from build123d import *

# Parameters (mm, degrees)
SM_BASE_FLANGE_1_DEPTH     = 1.5
SKETCH_6_R                 = 6.5
CUT_EXTRUDE_1_DEPTH        = 10
PATTERN_LINEAR_1_COUNT     = 2
PATTERN_LINEAR_1_PITCH     = 20
PATTERN_LINEAR_1_COL_COUNT = 2
PATTERN_LINEAR_1_COL_PITCH = 20
CHAMFER_1_SIZE             = 10


# Sheet-metal steps are written as plain solids
with BuildPart() as part:
    # Sketch 1 → Базовая кромка1 (new body)
    with BuildSketch(Plane.XY):
        Polygon((-50, 0), (50, 0), (50, 30), (0, 80), (-50, 30), align=None)
    extrude(amount=-SM_BASE_FLANGE_1_DEPTH)

    # Эскиз6 → Вырез-Вытянуть1 (cut)
    with BuildSketch(Plane.XY):
        with Locations((0, 32.623845661)):
            Circle(SKETCH_6_R)
    cut_extrude_1 = extrude(amount=-CUT_EXTRUDE_1_DEPTH, mode=Mode.SUBTRACT)

    # Линейный массив1: Вырез-Вытянуть1 ×2
    with Locations(*[(-i * PATTERN_LINEAR_1_PITCH, 0, 0) for i in range(1, PATTERN_LINEAR_1_COUNT)]):
        add(cut_extrude_1, mode=Mode.SUBTRACT)

    # Линейный массив1 col: Вырез-Вытянуть1 ×2
    with Locations(*[(i * PATTERN_LINEAR_1_COL_PITCH, 0, 0) for i in range(1, PATTERN_LINEAR_1_COL_COUNT)]):
        add(cut_extrude_1, mode=Mode.SUBTRACT)

    # Фаска1
    chamfer_1_edges = [part.edges().sort_by_distance(p)[0] for p in [
        (0, 80, -0.75),
    ]]
    chamfer(chamfer_1_edges, length=CHAMFER_1_SIZE)


solid = part.part
Geometry check sheet. Reference: the model listing, model coordinates, mm. Round coordinates to 2 decimals unless told otherwise and drop trailing zeros. Write each loop counter-clockwise with the first axis right and the second up, starting at its lowest first coordinate (ties: lowest second). Pieces come first, ordered by that corner, then holes. Notation, with made-up numbers: (2, -29.5) -> (50, -29.5) arc R34 cw to (50, 8.5) -> close; hole circle Ø1 at (72.25, -12.75). An arc over 180 degrees is marked (long way). One line per item, written item: value. Start each with the question number.
(1) Cross-section at A-A, the plane x = 0. Record the cut outline in (y, z), and give its area (3 significant figures).
(2) Cross-section at B-B, the plane z = -0.3. Record the cut outline in (x, y).
(3) Cross-section at C-C, the plane x = 20. Record the cut outline in (y, z), and give its area (3 significant figures).
(4) Cross-section at D-D, the plane y = 45.5. Record the cut outline in (x, z).
(5) Draft check along X on faces 1 (the cylindrical face through (-1.41, 26.28, -0.74)), 2 (the flat face through (29, 51, -1)), 3 (the cylindrical face through (14.84, 28.67, -0.74)), 4 (the flat face through (-1, 21, 0)). Enter one of: +X half, -X half, draft (parallel to the pull), parting line (faces both ways), or undercut.
(6) Go/stop test with flat-tipped pins: pin 1 Ø10.5 at (x, y) = (-20, 32.62) entering from +Z; pin 2 Ø8 at (x, y) = (35, 46) entering from -Z. Record where each tip stops, or that it passes through.
(7) Scan lines: line 1 (Y direction, x = 0, z = -0.75); line 2 (X direction, y = 37, z = -1.35); line 3 (X direction, y = 35, z = -0.95). Record each from-to range of solid material in increasing order. Write a range as [from, to].
Answer:
1. outline: (0, -1.5) -> (26.12, -1.5) -> (26.12, 0) -> (0, 0) -> close; (39.12, -1.5) -> (72.93, -1.5) -> (72.93, 0) -> (39.12, 0) -> close
1. area: 89.9 mm²
2. outline: (-50, 0) -> (50, 0) -> (50, 30) -> (7.07, 72.93) -> (-7.07, 72.93) -> (-50, 30) -> close; hole circle Ø13 at (-20, 32.62); hole circle Ø13 at (0, 32.62); hole circle Ø13 at (20, 32.62)
3. outline: (0, -1.5) -> (26.12, -1.5) -> (26.12, 0) -> (0, 0) -> close; (39.12, -1.5) -> (60, -1.5) -> (60, 0) -> (39.12, 0) -> close
3. area: 70.5 mm²
4. outline: (-34.5, -1.5) -> (34.5, -1.5) -> (34.5, 0) -> (-34.5, 0) -> close
5. face 1: undercut
5. face 2: +X half
5. face 3: undercut
5. face 4: draft
6. pin 1: through
6. pin 2: z = -1.5
7. line 1: [0, 26.12], [39.12, 72.93]
7. line 2: [-43, -24.81], [-15.19, -4.81], [4.81, 15.19], [24.81, 43]
7. line 3: [-45, -26.05], [-13.95, -6.05], [6.05, 13.95], [26.05, 45]
